```python
from build123d import *

# Parameters (mm, degrees)
SKETCH1_W           = 10
SKETCH1_H           = 25
SKETCH1_H_2         = 27
SKETCH1_W_2         = 14
SKETCH1_H_3         = 10
BOSS_EXTRUDE1_DEPTH = 1
SKETCH2_W           = 10
SKETCH2_H           = 1
BOSS_EXTRUDE2_DEPTH = 20


with BuildPart() as part:
    # Sketch1 → Boss-Extrude1 (new body)
    with BuildSketch(Plane(origin=(0, 0, 0), x_dir=(1, 0, 0), z_dir=(0, 1, 0))):
        with Locations((5, -39.5)):
            Rectangle(SKETCH1_W, SKETCH1_H)
        with Locations((5, -13.5)):
            Rectangle(SKETCH1_W, SKETCH1_H_2)
        with Locations((-7, -32)):
            Rectangle(SKETCH1_W_2, SKETCH1_H_3)
    extrude(amount=BOSS_EXTRUDE1_DEPTH)

    # Sketch2 → Boss-Extrude2 (add)
    with BuildSketch(Plane.XZ):
        with Locations((5, 51.5)):
            Rectangle(SKETCH2_W, SKETCH2_H)
    extrude(amount=-BOSS_EXTRUDE2_DEPTH)


solid = part.part
```
Input: part model. Units: mm. Frame: model coordinates. A direction names the side the tool comes from. Give positions to 0.01 mm unless a question says otherwise; leave off trailing zeros. Write each loop counter-clockwise with the first axis right and the second up, starting at its lowest first coordinate (ties: lowest second). Pieces come first, ordered by that corner, then holes. Notation, with made-up numbers: (-7.75, -12) - (31.25, -12) arc R26 cw to (31.25, 24) - close; hole circle Ø2 at (18.25, 62.5). An arc over 180 degrees is marked (long way). Write item = value, one per line. Start each with the question number.
1. Section query C-C, the plane z = 45.5. Output: boundary loops of the cut face in (x, y), then the cut area to 3 significant figures.
2. Section query A-A, the plane x = 4.75. Output: boundary loops of the cut face in (y, z), then the cut area to 3 significant figures.
3. Section query B-B, the plane y = 7. Output: boundary loops of the cut face in (x, z).
4. First-contact query: pin 1 Ø12 at (y, z) = (14, 47.5) entering from -X; pin 2 Ø4 at (x, z) = (2, 26.5) entering from -Y; pin 3 Ø4 at (x, y) = (-3.5, 16.5) entering from -Z; pin 4 Ø8 at (x, y) = (4, 9) entering from -Z. Flat tips, straight axial feed; report the tip coordinate or a pass-through.
5. Access query for faces 1 (the flat face through (3, 0, 26)), 2 (the flat face through (5, 10, 51)), 3 (the flat face through (-7.1, 0.5, 37)), 4 (the flat face through (5, 10, 52)), 5 (the flat face through (0, 0.5, 13.3)). Directions: +Z, -Z, +X, -X, +Y, -Y. A direction counts if a zero-diameter tool reaches every point of the face in a straight line with its end or side. Return the directions, or none.
6. Ray query, L1, parallel to Y at x = 3.75, z = 12.5; L2, parallel to Z at x = 7.75, y = 1.75. Return the intervals inside material, ascending.
Check sheet entries:
q1.outline = (0, 0) - (10, 0) - (10, 1) - (0, 1) - close
q1.area = 10.0 mm2
q2.outline = (0, 0) - (1, 0) - (1, 51) - (20, 51) - (20, 52) - (0, 52) - close
q2.area = 71.0 mm2
q3.outline = (0, 51) - (10, 51) - (10, 52) - (0, 52) - close
q4.pin_1 = 0
q4.pin_2 = 0
q4.pin_3 = through
q4.pin_4 = 51
q5.face_1 = +Z, -Z, +X, -X, -Y
q5.face_2 = -Z, +X, -X, +Y
q5.face_3 = +Z, -X, +Y, -Y
q5.face_4 = +Z, +X, -X, +Y, -Y
q5.face_5 = -Z, -X, +Y, -Y
q6.L1 = 0 to 1
q6.L2 = 51 to 52
